```python
from build123d import *

# Parameters (mm, degrees)
F0_W      = 61
F0_H      = 47
F0_R      = 1.45
F1_DEPTH  = 2
F3_W      = 48.5
F3_H      = 47
F3_R      = 5
F4_DEPTH  = 2
F5_W      = 48.5
F5_H      = 47
F5_R      = 10
F6_DEPTH  = 2
F8_W      = 61
F8_H      = 47
F8_R      = 5
F9_DEPTH  = 2
F11_W     = 61
F11_H     = 48.5
F12_DEPTH = 2
F14_W     = 61
F14_H     = 48.5
F15_DEPTH = 2


with BuildPart() as f1:
    # F0 (on Front) → F1 (new body)
    with BuildSketch(Plane.XZ):
        with Locations((30.5, 23.5)):
            Rectangle(F0_W, F0_H)
        Polygon((20, 5.5), (20, 7), (22, 7), (22, 5.5), (22, 4), (20, 4), align=None, mode=Mode.SUBTRACT)
        with Locations((30.5, 5.5)):
            Circle(F0_R, mode=Mode.SUBTRACT)
    extrude(amount=F1_DEPTH)

    # F3 (on offset) → F4 (join)
    with BuildSketch(Plane.YZ.offset(61)):
        with Locations((-24.25, 23.5)):
            Rectangle(F3_W, F3_H)
        with Locations((-38.5, 10)):
            Circle(F3_R, mode=Mode.SUBTRACT)
        Polygon((-34.25, 37), (-24.25, 37), (-14.25, 37), (-14.25, 17), (-34.25, 17), align=None, mode=Mode.SUBTRACT)
    extrude(amount=-F4_DEPTH)

    # F5 (on Right) → F6 (join)
    with BuildSketch(Plane.YZ):
        with Locations((-24.25, 23.5)):
            Rectangle(F5_W, F5_H)
        with Locations((-24.25, 23.5)):
            Circle(F5_R, mode=Mode.SUBTRACT)
    extrude(amount=F6_DEPTH)

    # F8 (on offset) → F9 (join)
    with BuildSketch(Plane.XZ.offset(48.5)):
        with Locations((30.5, 23.5)):
            Rectangle(F8_W, F8_H)
        with Locations((15.25, 23.5)):
            Circle(F8_R, mode=Mode.SUBTRACT)
        with Locations((45.75, 23.5)):
            Circle(F8_R, mode=Mode.SUBTRACT)
    extrude(amount=-F9_DEPTH)

    # F11 (on offset) → F12 (join)
    with BuildSketch(Plane.XY.offset(47)):
        with Locations((30.5, -24.25)):
            Rectangle(F11_W, F11_H)
    extrude(amount=-F12_DEPTH)

    # F14 (on offset) → F15 (join)
    with BuildSketch(Plane(origin=(0, 0, 0), x_dir=(1, 0, 0), z_dir=(0, 0, -1))):
        with Locations((30.5, 24.25)):
            Rectangle(F14_W, F14_H)
    extrude(amount=-F15_DEPTH)


solid = f1.part
```
For this review, take the finished solid that the model builds, in its own axes (mm). A direction names the side the tool comes from. Give positions to 0.01 mm unless a question says otherwise; leave off trailing zeros. Order: outer loops, then holes, each group sorted by start corner. A loop starts at its lowest first (then second) coordinate and runs counter-clockwise, first axis right, second up.
1) Wall thickness on line 1 (Z direction, x = 17, y = -17); line 2 (Y direction, x = 31.5, z = 15); line 3 (X direction, y = -38, z = 30.5): over which ranges is each line inside the solid? List them lowest first.
2) For faces 1 (the face through (21, -1, 7)), 2 (the face through (30, -46.5, 24)), 3 (the face through (17.557, -47.514, 19.064)), list the 3-axis set-ups (+Z, -Z, +X, -X, +Y, -Y) from which the entire face can be reached by the end or side of a thin tool; tool diameter is ignored.
3) Take a section at C-C (x = 27). Give the boundary of the cut face in (y, z).
4) Take a section at D-D (z = 43). Give the boundary of the cut face in (x, y).
5) Take a section at B-B (z = 23.5). Give the boundary of the cut face in (x, y).
6) The part is to be moulded in two halves that separate along Z. For faces 4 (the face through (30, -48.5, 23)), 5 (the face through (30, -25, 47)), 6 (the face through (30, -25, 2)), say which applies: released by +Z, released by -Z, zero draft, split by the parting line, or undercut.
7) Take a section at A-A (y = -24.25). Give the boundary of the cut face in (x, z).
8) Insertion check: pin 1 (1.6 mm diameter, centred on y = -1, z = 5.5, fed in from -X); pin 2 (9 mm diameter, centred on x = 45.75, z = 23.5, fed in from -Y). Each pin has a flat end and moves straight along its axis. Give the tip position at first contact, or say it passes through.
Derived:
1. line 1: z = 0 to 2, 45 to 47
1. line 2: y = -48.5 to -46.5, -2 to 0
1. line 3: x = 0 to 2, 59 to 61
2. face 1: +Y
2. face 2: none
2. face 3: -Y
3. outline: (-48.5, 0) - (0, 0) - (0, 47) - (-48.5, 47) - close; hole (-46.5, 2) - (-2, 2) - (-2, 45) - (-46.5, 45) - close
4. outline: (0, -48.5) - (61, -48.5) - (61, 0) - (0, 0) - close; hole (2, -46.5) - (59, -46.5) - (59, -2) - (2, -2) - close
5. outline: (0, -48.5) - (10.25, -48.5) - (10.25, -46.5) - (2, -46.5) - (2, -34.25) - (0, -34.25) - close; (0, -14.25) - (2, -14.25) - (2, -2) - (59, -2) - (59, -14.25) - (61, -14.25) - (61, 0) - (0, 0) - close; (20.25, -48.5) - (40.75, -48.5) - (40.75, -46.5) - (20.25, -46.5) - close; (50.75, -48.5) - (61, -48.5) - (61, -34.25) - (59, -34.25) - (59, -46.5) - (50.75, -46.5) - close
6. face 4: zero draft
6. face 5: released by +Z
6. face 6: undercut
7. outline: (0, 0) - (61, 0) - (61, 17) - (59, 17) - (59, 2) - (2, 2) - (2, 13.5) - (0, 13.5) - close; (0, 33.5) - (2, 33.5) - (2, 45) - (59, 45) - (59, 37) - (61, 37) - (61, 47) - (0, 47) - close
8. pin 1: stops at x = 0
8. pin 2: stops at y = -2
